from build123d import *

# Parameters (mm, degrees)
F0_W     = 62.23
F0_H     = 9.525
F0_R     = 1.593097
F0_R_2   = 1.5875
F0_R_3   = 1.58325
F1_DEPTH = 1.89738


with BuildPart() as f1:
    # F0 (on Front) → F1 (new body)
    with BuildSketch(Plane.XZ):
        with Locations((-9.849542, 15.549641)):
            Rectangle(F0_W, F0_H)
        with Locations((-32.074542, 15.549641)):
            Circle(F0_R, mode=Mode.SUBTRACT)
        with Locations((-23.184542, 15.549641)):
            Circle(F0_R_2, mode=Mode.SUBTRACT)
        with Locations((-14.294542, 15.549641)):
            Circle(F0_R_3, mode=Mode.SUBTRACT)
        with Locations((-5.404542, 15.549641)):
            Circle(F0_R, mode=Mode.SUBTRACT)
        with Locations((3.485458, 15.549641)):
            Circle(F0_R_2, mode=Mode.SUBTRACT)
        with Locations((12.375458, 15.552476)):
            Circle(F0_R_3, mode=Mode.SUBTRACT)
    extrude(amount=F1_DEPTH)


solid = f1.part
Read the model definition and answer for the solid it produces. Units are mm, in the model's axes. Round coordinates to 2 decimals unless told otherwise and drop trailing zeros. Write each loop counter-clockwise with the first axis right and the second up, starting at its lowest first coordinate (ties: lowest second). Pieces come first, ordered by that corner, then holes.
Q1. Find section B-B on x = -24. Determine the outline of the cut face in (y, z).
Values:
outline: (-1.9, 10.79) - (0, 10.79) - (0, 14.19) - (-1.9, 14.19) - close; (-1.9, 16.91) - (0, 16.91) - (0, 20.31) - (-1.9, 20.31) - close
Q2. A flat-ended cylindrical pin translates along its axis: P1, Ø1.9, axis at x = -14.29, z = 15.55, coming from the -Y side (1 decimal). Find the tip coordinate at first contact, or state that the pin passes through.
Values:
P1: passes through
Q3. Find section A-A on z = 14.5. Determine the outline of the cut face in (x, y).
Values:
outline: (-40.96, -1.9) - (-33.27, -1.9) - (-33.27, 0) - (-40.96, 0) - close; (-30.88, -1.9) - (-24.38, -1.9) - (-24.38, 0) - (-30.88, 0) - close; (-21.99, -1.9) - (-15.48, -1.9) - (-15.48, 0) - (-21.99, 0) - close; (-13.11, -1.9) - (-6.6, -1.9) - (-6.6, 0) - (-13.11, 0) - close; (-4.21, -1.9) - (2.29, -1.9) - (2.29, 0) - (-4.21, 0) - close; (4.68, -1.9) - (11.19, -1.9) - (11.19, 0) - (4.68, 0) - close; (13.56, -1.9) - (21.27, -1.9) - (21.27, 0) - (13.56, 0) - close
Q4. The mould has two halves that part along Z. Classify faces 1 (the face through (-14.5, -0.94, 17.12)), 2 (the face through (-23.391, -0.935, 17.124)), 3 (the face through (-10, -1, 10.787)), 4 (the face through (-10, -1, 20.312)): released by +Z, released by -Z, zero draft, split by the parting line, or undercut.
Values:
face 1: undercut
face 2: undercut
face 3: released by -Z
face 4: released by +Z
Q5. Find section D-D on x = -31.5. Determine the outline of the cut face in (y, z), and give its area (3 significant figures).
Values:
outline: (-1.9, 10.79) - (0, 10.79) - (0, 14.06) - (-1.9, 14.06) - close; (-1.9, 17.04) - (0, 17.04) - (0, 20.31) - (-1.9, 20.31) - close
area: 12.4 mm2
Q6. Straight lines are drawn through the part: line 1 (Z direction, x = -31, y = -1.65); line 2 (Z direction, x = -33, y = -1.5). For each, find the intervals that lie inside material, in ascending order.
Values:
line 1: z = 10.79 to 14.37, 16.73 to 20.31
line 2: z = 10.79 to 14.25, 16.85 to 20.31
Q7. Find section C-C on y = -1.25. Determine the outline of the cut face in (x, z) (1 decimal).
Values:
outline: (-41, 10.8) - (21.3, 10.8) - (21.3, 20.3) - (-41, 20.3) - close; hole circle Ø3.2 at (-32.1, 15.5); hole circle Ø3.2 at (-23.2, 15.5); hole circle Ø3.2 at (-14.3, 15.5); hole circle Ø3.2 at (-5.4, 15.5); hole circle Ø3.2 at (3.5, 15.5); hole circle Ø3.2 at (12.4, 15.6)
